Can you work these out from the model? Positions are in its coordinate system, mm. Face numbers are marked on the shaded views. A direction names the side the tool comes from. Give positions to 0.01 mm unless a question says otherwise; leave off trailing zeros. Loops run counter-clockwise (first coordinate to the right, second up) from the corner with the lowest first, then second, coordinate; pieces in that order, holes last. Notation, with made-up numbers: M 16.5,34.5 L 26.5,34.5 A22 cw 26.5,40.5 Z; hole C -16,-35.5 d6. An arc over 180 degrees is marked long. Put each result on its own line as item: value. Start each with the question number.
1) Imagine slicing it at A-A (x = 8). Write out the boundary of the cut face in (y, z), then the cut area to 3 significant figures.
2) Imagine slicing it at C-C (y = -27). Write out the boundary of the cut face in (x, z), then the cut area to 3 significant figures.
3) For the marked faces 1, 2 and 3, which set-ups out of +Z, -Z, +X, -X, +Y, -Y let a thin tool reach every point of the face, with its end or its side?
4) Please list where these lines run through material, in increasing order: line 1 along X through (y, z) = (31.5, 5); line 2 along X through (y, z) = (-22, 3.75). Write a range as from..to.
5) Imagine slicing it at B-B (z = 3.25). Write out the boundary of the cut face in (x, y), then the cut area to 3 significant figures.
6) For P1, Ø1, axis at y = -12, z = 3.5, coming from the -X side; P2, Ø3, axis at y = 15, z = 3.5, coming from the +X side; P3, Ø3, axis at y = 22.5, z = 4.5, coming from the +X side, each with a flat end and sliding along its axis, tell me the tip position at first contact or that it passes through.
7) Imagine slicing it at D-D (x = 13). Write out the boundary of the cut face in (y, z).
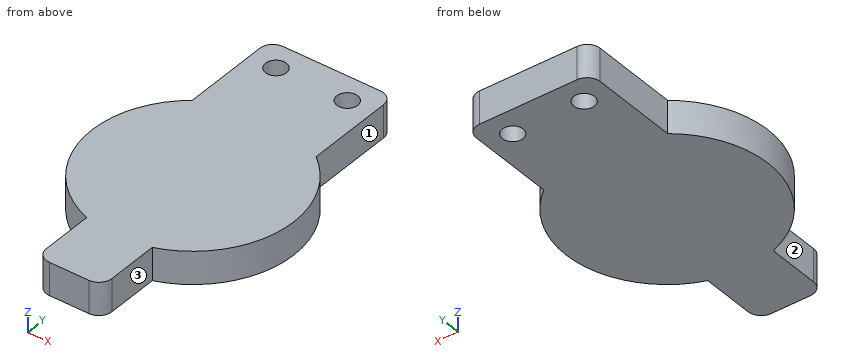
from build123d import *

# Parameters (mm, degrees)
SKETCH1_R           = 2.032
BOSS_EXTRUDE1_DEPTH = 6.35
FILLET1_R           = 2.54


with BuildPart() as part:
    # Sketch1 → Boss-Extrude1 (new body)
    with BuildSketch(Plane.XY):
        with BuildLine():
            ThreePointArc((6.35, -18.498455719), (0, -19.558), (-6.35, -18.498455719))
            Line((-6.35, -18.498455719), (-6.35, -31.198455719))
            Line((-6.35, -31.198455719), (6.35, -31.198455719))
            Line((6.35, -31.198455719), (6.35, -18.498455719))
        make_face()
        with BuildLine():
            Line((-11.994797213, 34.995050133), (-11.994797213, 15.447983811))
            ThreePointArc((-11.994797213, 15.447983811), (-19.293083875, -3.208158134), (-6.35, -18.498455719))
            Line((-6.35, -18.498455719), (6.35, -18.498455719))
            ThreePointArc((6.35, -18.498455719), (19.293083875, -3.208158134), (11.994797213, 15.447983811))
            Line((11.994797213, 15.447983811), (11.994797213, 34.995050133))
            Line((11.994797213, 34.995050133), (-11.994797213, 34.995050133))
        make_face()
        with Locations((-6.914797213, 29.915050133)):
            Circle(SKETCH1_R, mode=Mode.SUBTRACT)
        with Locations((6.914797213, 29.915050133)):
            Circle(SKETCH1_R, mode=Mode.SUBTRACT)
        with BuildLine():
            Line((6.35, -18.498455719), (-6.35, -18.498455719))
            ThreePointArc((-6.35, -18.498455719), (0, -19.558), (6.35, -18.498455719))
        make_face()
    extrude(amount=BOSS_EXTRUDE1_DEPTH)

    # Fillet1
    fillet1_edges = [part.edges().sort_by_distance(p)[0] for p in [
        (6.35, -31.198455719, 3.175),
        (-6.35, -31.198455719, 3.175),
        (11.994797213, 34.995050133, 3.175),
        (-11.994797213, 34.995050133, 3.175),
    ]]
    fillet(fillet1_edges, radius=FILLET1_R)


solid = part.part
Recorded:
1. outline: M -17.85,0 L 28.2,0 L 28.2,6.35 L -17.85,6.35 Z; M 31.63,0 L 35,0 L 35,6.35 L 31.63,6.35 Z
1. area: 314 mm²
2. outline: M -6.35,0 L 6.35,0 L 6.35,6.35 L -6.35,6.35 Z
2. area: 80.6 mm²
3. face 1: +Z, -Z, +X, +Y
3. face 2: +Z, -Z, -X, -Y
3. face 3: +Z, -Z, +X, -Y
4. line 1: -11.99..-8.19, -5.64..5.64, 8.19..11.99
4. line 2: -6.35..6.35
5. outline: M -11.99,15.45 A19.56 ccw -6.35,-18.5 L -6.35,-28.66 A2.54 ccw -3.81,-31.2 L 3.81,-31.2 A2.54 ccw 6.35,-28.66 L 6.35,-18.5 A19.56 ccw 11.99,15.45 L 11.99,32.46 A2.54 ccw 9.45,35 L -9.45,35 A2.54 ccw -11.99,32.46 Z; hole C -6.91,29.92 d4.06; hole C 6.91,29.92 d4.06
5. area: 1,720 mm²
6. P1: x = -15.82
6. P2: x = 14.15
6. P3: x = 11.99
7. outline: M -14.61,0 L 14.61,0 L 14.61,6.35 L -14.61,6.35 Z
